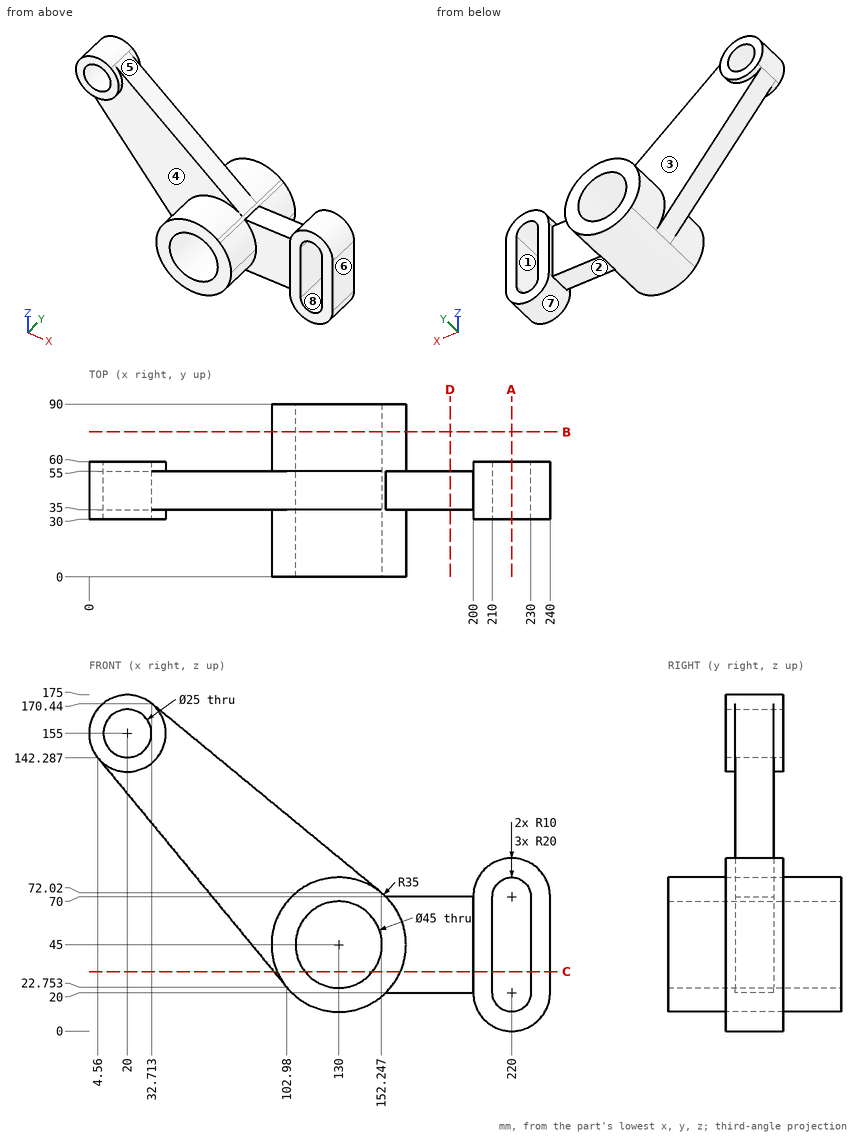
For this review, use the dimensioned drawing (mm, ordinates from the lowest corner) and the shaded views. A direction names the side the tool comes from. Give positions to 0.01 mm unless a question says otherwise; leave off trailing zeros. Write each loop counter-clockwise with the first axis right and the second up, starting at its lowest first coordinate (ties: lowest second). Pieces come first, ordered by that corner, then holes. Notation, with made-up numbers: M 31.5,-39 L 69.5,-39 A24 ccw 69.5,-21 Z; hole C 53,42.25 d9. An arc over 180 degrees is marked long. Answer as a JSON object with one key per item and string values. Group by question number.
1) We need section D-D (x = 188). Give the boundary of the cut face in (y, z), and give its area (3 significant figures).
2) Clearance check with flat-ended pins moving along their axes: pin 1 Ø12 at (y, z) = (75.5, 49.5) entering from +X; pin 2 Ø1 at (x, z) = (59.5, 137) entering from +Y; pin 3 Ø1.5 at (x, z) = (76.5, 106) entering from -Y. State where each tip first meets the part, or that it passes through.
3) We need section C-C (z = 31). Give the boundary of the cut face in (x, y).
4) We need section B-B (y = 75.5). Give the boundary of the cut face in (x, z) (1 decimal), and give its area (3 significant figures).
5) We need section A-A (x = 220). Give the boundary of the cut face in (y, z), and give its area (3 significant figures).
6) Mouldability with a two-part tool opening along Z and no side actions: class the marked faces 1, 2 and 3 as released by +Z, released by -Z, zero draft, split by the parting line, or undercut.
7) For line 1 along X through (y, z) = (43, 42) (1 decimal); line 2 along Z through (x, y) = (130, 60); line 3 along X through (y, z) = (47.5, 51.5), list the stretches that pass through material, from the lowest coordinate up.
8) Tool access review of the marked faces 4, 5, 6, 7 and 8: name each direction out of +Z, -Z, +X, -X, +Y, -Y from which nothing blocks a thin tool from reaching the whole face with its end or side.
Answer key:
{
 "1": {"outline": "M 35,20 L 55,20 L 55,70 L 35,70 Z", "area": "1,000 mm²"},
 "2": {"pin 1": "stops at x = 165", "pin 2": "stops at y = 55", "pin 3": "stops at y = 35"},
 "3": {"outline": "M 96.19,35 L 97.92,35 L 97.92,0 L 112.39,0 L 112.39,90 L 97.92,90 L 97.92,55 L 96.19,55 Z; M 147.61,0 L 162.08,0 L 162.08,35 L 200,35 L 200,30 L 210,30 L 210,60 L 200,60 L 200,55 L 162.08,55 L 162.08,90 L 147.61,90 Z; M 230,30 L 240,30 L 240,60 L 230,60 Z"},
 "4": {"outline": "M 103,22.8 A35 ccw 154.5,20 A35 ccw 165,45 A35 ccw 154.5,70 A35 ccw 152.2,72 A35 ccw Z; hole C 130,45 d45", "area": "2,260 mm²"},
 "5": {"outline": "M 30,0 L 60,0 L 60,10 L 30,10 Z; M 30,80 L 60,80 L 60,90 L 30,90 Z", "area": "600 mm²"},
 "6": {"face 1": "undercut", "face 2": "released by -Z", "face 3": "zero draft"},
 "7": {"line 1": "x = 87.1 to 107.7, 152.3 to 210, 230 to 240", "line 2": "z = 10 to 22.5, 67.5 to 80", "line 3": "x = 79.31 to 108.46, 151.54 to 210, 230 to 240"},
 "8": {"face 4": "-Y", "face 5": "+Z, +Y, -Y", "face 6": "+Z, -Z, +X, +Y, -Y", "face 7": "-Z, +Y, -Y", "face 8": "+Y, -Y"}
}
